Could you check a few things on this model? Use its own coordinates, in mm. A direction names the side the tool comes from. Give positions to 0.01 mm unless a question says otherwise; leave off trailing zeros. Write each loop counter-clockwise with the first axis right and the second up, starting at its lowest first coordinate (ties: lowest second). Pieces come first, ordered by that corner, then holes. Notation, with made-up numbers: M 18,55 L 39,55 A21 ccw 39,80 Z; hole C -27,-35.75 d1. An arc over 180 degrees is marked long. One line per item, written item: value.
```python
from build123d import *

# Parameters (mm, degrees)
F1_DEPTH = 620


with BuildPart() as f1:
    # F0 (on Front) → F1 (new body)
    with BuildSketch(Plane.XZ):
        with BuildLine():
            Line((14, 30), (-14, 30))
            ThreePointArc((-14, 30), (-18.242641, 28.242641), (-20, 24))
            Line((-20, 24), (-20, -24))
            ThreePointArc((-20, -24), (-18.242641, -28.242641), (-14, -30))
            Line((-14, -30), (14, -30))
            ThreePointArc((14, -30), (18.242641, -28.242641), (20, -24))
            Line((20, -24), (20, 24))
            ThreePointArc((20, 24), (18.242641, 28.242641), (14, 30))
        make_face()
        with BuildLine():
            Line((-17, -24), (-17, 24))
            ThreePointArc((-17, 24), (-16.12132, 26.12132), (-14, 27))
            Line((-14, 27), (14, 27))
            ThreePointArc((14, 27), (16.12132, 26.12132), (17, 24))
            Line((17, 24), (17, -24))
            ThreePointArc((17, -24), (16.12132, -26.12132), (14, -27))
            Line((14, -27), (-14, -27))
            ThreePointArc((-14, -27), (-16.12132, -26.12132), (-17, -24))
        make_face(mode=Mode.SUBTRACT)
    extrude(amount=F1_DEPTH)


solid = f1.part
```
1) If we section it at B-B, the plane z = 19: Write out the boundary of the cut face in (x, y), then the cut area to 3 significant figures.
Outcome:
outline: M -20,-620 L -17,-620 L -17,0 L -20,0 Z; M 17,-620 L 20,-620 L 20,0 L 17,0 Z
area: 3,720 mm^2
2) On a 3-axis mill with a long thin cutter (end or side, diameter ignored), from which of +Z, -Z, +X, -X, +Y, -Y can I reach the whole of each face in a straight line? I mean faces 1 (the face through (-17, -306, 0)), 2 (the face through (20, -306, 0)). Say none if no direction works.
Outcome:
face 1: +Y, -Y
face 2: +Z, -Z, +X, +Y, -Y
3) If we section it at C-C, the plane y = -176: Write out the boundary of the cut face in (x, z).
Outcome:
outline: M -20,-24 A6 ccw -14,-30 L 14,-30 A6 ccw 20,-24 L 20,24 A6 ccw 14,30 L -14,30 A6 ccw -20,24 Z; hole M -17,-24 A3 ccw -14,-27 L 14,-27 A3 ccw 17,-24 L 17,24 A3 ccw 14,27 L -14,27 A3 ccw -17,24 Z
4) Please list where these lines run through material, in increasing order: L1, parallel to X at y = -473, z = -21.5; L2, parallel to Z at x = -7, y = -552.5; L3, parallel to Z at x = -15, y = -592. Write a range as from..to.
Outcome:
L1: x = -20..-17, 17..20
L2: z = -30..-27, 27..30
L3: z = -29.92..-26.83, 26.83..29.92
5) We'd pull the mould along Z, two halves only. Please class faces 3 (the face through (0, -306, 27)), 4 (the face through (18, 0, 0)), 5 (the face through (0, -306, 30)): pulls with the +Z half, pulls with the -Z half, needs draft (parallel to the pull), parting line crosses it, or undercut.
Outcome:
face 3: undercut
face 4: needs draft
face 5: pulls with the +Z half
6) If we section it at A-A, the plane x = -2: Write out the boundary of the cut face in (y, z), then the cut area to 3 significant figures.
Outcome:
outline: M -620,-30 L 0,-30 L 0,-27 L -620,-27 Z; M -620,27 L 0,27 L 0,30 L -620,30 Z
area: 3,720 mm^2
